Geometry check sheet. Reference: the model listing, model coordinates, mm. A direction names the side the tool comes from. Round coordinates to 2 decimals unless told otherwise and drop trailing zeros. Order: outer loops, then holes, each group sorted by start corner. A loop starts at its lowest first (then second) coordinate and runs counter-clockwise, first axis right, second up.
(1) Draft check along Z on faces 1 (the face through (47.5, 2.5, 35.1)), 2 (the face through (-0.7, 2.5, 50)), 3 (the face through (-1, 5, 22)). Enter one of: pulls with the +Z half, pulls with the -Z half, needs draft (parallel to the pull), parting line crosses it, or undercut.
(2) Cross-section at D-D on x = -33. Enter the section's corners in (y, z), and give its area (3 significant figures).
(3) Cross-section at A-A on x = 0. Enter the section's corners in (y, z).
(4) Gauge pin test, flat ends, axial feed: P1, Ø1.5, axis at x = 23, y = 1.5, coming from the +Z side; P2, Ø2.5, axis at x = 0, z = 43, coming from the -Y side. Record the tip position at first contact, or that the pin passes through.
(5) Thickness scan on L1, parallel to Z at x = 6.5, y = 3.4; L2, parallel to Z at x = 4, y = 2. Record the ranges inside material, lowest first.
(6) Set-up check for faces 4 (the face through (50, 2, 18)), 5 (the face through (-25, 3, -2.5)): record each of +Z, -Z, +X, -X, +Y, -Y from which the full face is reachable in a straight line by a thin tool's end or side.
(7) Cross-section at C-C on y = 1. Enter the section's corners in (x, z).
(8) Cross-section at B-B on z = 35. Enter the section's corners in (x, y).
from build123d import *

# Parameters (mm, degrees)
BOSS_EXTRUDE1_DEPTH = 5
CUT_EXTRUDE1_REACH  = 72.887
CUT_EXTRUDE2_REACH  = 72.887
SKETCH3_R           = 2


with BuildPart() as part:
    # Sketch1 → Boss-Extrude1 (new body)
    with BuildSketch(Plane(origin=(0, 0, 0), x_dir=(1, 0, 0), z_dir=(0, 1, 0))):
        with BuildLine():
            Line((50, -40), (50, 5))
            Line((50, 5), (-50, 5))
            Line((-50, 5), (-50, -40))
            ThreePointArc((-50, -40), (0, -50), (50, -40))
        make_face()
    extrude(amount=BOSS_EXTRUDE1_DEPTH)

    # Sketch2 → Cut-Extrude1 (cut, up to next)
    with BuildSketch(Plane(origin=(0, 5, 0), x_dir=(1, 0, 0), z_dir=(0, 1, 0)), mode=Mode.PRIVATE) as cut_extrude1_sk1:
        with BuildLine():
            Line((-45, -32.5), (-5, -32.5))
            ThreePointArc((-5, -32.5), (-2.5, -35), (-5, -37.5))
            Line((-5, -37.5), (-45, -37.5))
            ThreePointArc((-45, -37.5), (-47.5, -35), (-45, -32.5))
        make_face()
    cut_extrude1_tool1 = extrude(cut_extrude1_sk1.sketch, amount=-CUT_EXTRUDE1_REACH, mode=Mode.PRIVATE) & part.part
    # Sketch2 → Cut-Extrude1 (cut, up to next)
    with BuildSketch(Plane(origin=(0, 5, 0), x_dir=(1, 0, 0), z_dir=(0, 1, 0)), mode=Mode.PRIVATE) as cut_extrude1_sk2:
        with BuildLine():
            Line((-45, 2.5), (-5, 2.5))
            ThreePointArc((-5, 2.5), (-2.5, 0), (-5, -2.5))
            Line((-5, -2.5), (-45, -2.5))
            ThreePointArc((-45, -2.5), (-47.5, 0), (-45, 2.5))
        make_face()
    cut_extrude1_tool2 = extrude(cut_extrude1_sk2.sketch, amount=-CUT_EXTRUDE1_REACH, mode=Mode.PRIVATE) & part.part
    cut_extrude1_1 = cut_extrude1_tool1.solids().sort_by_distance((-25, 5, 35))[0]
    add(cut_extrude1_1, mode=Mode.SUBTRACT)
    cut_extrude1_2 = cut_extrude1_tool2.solids().sort_by_distance((-25, 5, 0))[0]
    add(cut_extrude1_2, mode=Mode.SUBTRACT)
    cut_extrude1 = cut_extrude1_1 + cut_extrude1_2  # Cut-Extrude1 as one shape, for the pattern or mirror that repeats it

    # Mirror1: Cut-Extrude1 across plane
    add(cut_extrude1.mirror(Plane(origin=(0, 0, 0), x_dir=(0, 0, 1), z_dir=(1, 0, 0))), mode=Mode.SUBTRACT)

    # Sketch3 → Cut-Extrude2 (cut, up to next)
    with BuildSketch(Plane(origin=(0, 5, 0), x_dir=(1, 0, 0), z_dir=(0, 1, 0)), mode=Mode.PRIVATE) as cut_extrude2_sk1:
        with Locations(Location((0, -43, 0), (0, 0, 270))):
            Circle(SKETCH3_R)
    cut_extrude2_tool1 = extrude(cut_extrude2_sk1.sketch, amount=-CUT_EXTRUDE2_REACH, mode=Mode.PRIVATE) & part.part
    add(cut_extrude2_tool1.solids().sort_by_distance((0, 5, 43))[0], mode=Mode.SUBTRACT)


solid = part.part
Found:
1. face 1: undercut
1. face 2: pulls with the +Z half
1. face 3: needs draft
2. outline: (0, -5) - (5, -5) - (5, -2.5) - (0, -2.5) - close; (0, 2.5) - (5, 2.5) - (5, 32.5) - (0, 32.5) - close; (0, 37.5) - (5, 37.5) - (5, 45.74) - (0, 45.74) - close
2. area: 204 mm2
3. outline: (0, -5) - (5, -5) - (5, 41) - (0, 41) - close; (0, 45) - (5, 45) - (5, 50) - (0, 50) - close
4. P1: stops at z = 48.08
4. P2: passes through
5. L1: z = -5 to -2.5, 2.5 to 32.5, 37.5 to 49.84
5. L2: z = -5 to -2.29, 2.29 to 32.71, 37.29 to 49.94
6. face 4: +Z, -Z, +X, +Y, -Y
6. face 5: +Y, -Y
7. outline: (-50, -5) - (50, -5) - (50, 40) arc R130 ccw to (-50, 40) - close; hole (-45, -2.5) - (-5, -2.5) arc R2.5 ccw to (-5, 2.5) - (-45, 2.5) arc R2.5 ccw to start; hole (-45, 32.5) - (-5, 32.5) arc R2.5 ccw to (-5, 37.5) - (-45, 37.5) arc R2.5 ccw to start; hole circle Ø4 at (0, 43); hole (5, -2.5) - (45, -2.5) arc R2.5 ccw to (45, 2.5) - (5, 2.5) arc R2.5 ccw to start; hole (5, 32.5) - (45, 32.5) arc R2.5 ccw to (45, 37.5) - (5, 37.5) arc R2.5 ccw to start
8. outline: (-50, 0) - (-47.5, 0) - (-47.5, 5) - (-50, 5) - close; (-2.5, 0) - (2.5, 0) - (2.5, 5) - (-2.5, 5) - close; (47.5, 0) - (50, 0) - (50, 5) - (47.5, 5) - close
